```python
from build123d import *

# Parameters (mm, degrees)
SKETCH_2_W          = 65
SKETCH_2_H          = 29
EXTRUDE_1_DEPTH     = 24
FILLET_1_R          = 2
SKETCH_3_R          = 1
CUT_EXTRUDE_1_DEPTH = 6
SKETCH_4_R          = 8
EXTRUDE_2_DEPTH     = 1
FILLET_2_R          = 1
SKETCH_5_R          = 4
EXTRUDE_3_DEPTH     = 6
SKETCH_6_R          = 1
CUT_EXTRUDE_2_DEPTH = 6
EXTRUDE_START       = 1
SKETCH_7_R          = 8
EXTRUDE_4_DEPTH     = 1
FILLET_3_R          = 1
SKETCH_8_R          = 3.5
EXTRUDE_5_DEPTH     = 0.3
SKETCH_9_R          = 3
EXTRUDE_6_DEPTH     = 5.5
SKETCH_10_R         = 1
CUT_EXTRUDE_3_DEPTH = 5.5
SKETCH_11_W         = 6.5
SKETCH_11_H         = 3
EXTRUDE_7_DEPTH     = 1
SKETCH_12_R         = 1.5
CUT_EXTRUDE_4_DEPTH = 6


with BuildPart() as part:
    # ｽｹｯﾁ2 → ﾎﾞｽ - 押し出し1 (new, symmetric)
    with BuildSketch(Plane(origin=(0, 0, 0), x_dir=(1, 0, 0), z_dir=(0, 1, 0))):
        Rectangle(SKETCH_2_W, SKETCH_2_H)
    extrude(amount=EXTRUDE_1_DEPTH, both=True)

    # ﾌｨﾚｯﾄ1
    fillet_1_edges = [part.edges().sort_by_distance(p)[0] for p in [
        (32.5, 0, 14.5),
        (-32.5, 0, 14.5),
        (-32.5, 0, -14.5),
        (32.5, 0, -14.5),
    ]]
    fillet(fillet_1_edges, radius=FILLET_1_R)

    # ｽｹｯﾁ3 → ｶｯﾄ - 押し出し1 (cut)
    with BuildSketch(Plane(origin=(0, 24, 0), x_dir=(1, 0, 0), z_dir=(0, 1, 0))):
        with Locations(Location((-29.5, 0, 0), (0, 0, 270))):
            Circle(SKETCH_3_R)
        with Locations(Location((-17.5, -13, 0), (0, 0, 270))):
            Circle(SKETCH_3_R)
        with Locations(Location((-17.5, 13, 0), (0, 0, 90))):
            Circle(SKETCH_3_R)
    extrude(amount=-CUT_EXTRUDE_1_DEPTH, mode=Mode.SUBTRACT)

    # ｽｹｯﾁ4 → ﾎﾞｽ - 押し出し2 (add)
    with BuildSketch(Plane(origin=(0, 24, 0), x_dir=(1, 0, 0), z_dir=(0, 1, 0))):
        with Locations(Location((20, 0, 0), (0, 0, 270))):
            Circle(SKETCH_4_R)
    extrude(amount=EXTRUDE_2_DEPTH)

    # ﾌｨﾚｯﾄ2
    fillet_2_edges = [part.edges().sort_by_distance(p)[0] for p in [
        (20, 24, -8),
    ]]
    fillet(fillet_2_edges, radius=FILLET_2_R - 0.0001)  # a hair under: the kernel refuses the full size

    # ｽｹｯﾁ5 → ﾎﾞｽ - 押し出し3 (add)
    with BuildSketch(Plane(origin=(0, 25, 0), x_dir=(1, 0, 0), z_dir=(0, 1, 0))):
        with Locations(Location((20, 0, 0), (0, 0, 270))):
            Circle(SKETCH_5_R)
    extrude(amount=EXTRUDE_3_DEPTH)

    # ｽｹｯﾁ6 → ｶｯﾄ - 押し出し2 (cut)
    with BuildSketch(Plane.XZ.offset(24)):
        with Locations(Location((-29.5, 13, 0), (0, 0, 270))):
            Circle(SKETCH_6_R)
        with Locations(Location((-29.5, -13, 0), (0, 0, 90))):
            Circle(SKETCH_6_R)
        with Locations(Location((29.5, -13, 0), (0, 0, 270))):
            Circle(SKETCH_6_R)
        with Locations(Location((29.5, 13, 0), (0, 0, 90))):
            Circle(SKETCH_6_R)
        with Locations(Location((-5.5, 13, 0), (0, 0, 270))):
            Circle(SKETCH_6_R)
        with Locations(Location((-5.5, -13, 0), (0, 0, 90))):
            Circle(SKETCH_6_R)
    extrude(amount=-CUT_EXTRUDE_2_DEPTH, mode=Mode.SUBTRACT)

    # ｽｹｯﾁ7 → ﾎﾞｽ - 押し出し4 (add)
    with BuildSketch(Plane.XZ.offset(24).offset(EXTRUDE_START)):
        with Locations(Location((20, 0, 0), (0, 0, 90))):
            Circle(SKETCH_7_R)
    extrude(amount=-EXTRUDE_4_DEPTH)

    # ﾌｨﾚｯﾄ3
    fillet_3_edges = [part.edges().sort_by_distance(p)[0] for p in [
        (20, -24, -8),
    ]]
    fillet(fillet_3_edges, radius=FILLET_3_R - 0.0001)  # a hair under: the kernel refuses the full size

    # ｽｹｯﾁ8 → ﾎﾞｽ - 押し出し5 (add)
    with BuildSketch(Plane.XZ.offset(25)):
        with Locations(Location((20, 0, 0), (0, 0, 270))):
            Circle(SKETCH_8_R)
    extrude(amount=EXTRUDE_5_DEPTH)

    # ｽｹｯﾁ9 → ﾎﾞｽ - 押し出し6 (add)
    with BuildSketch(Plane.XZ.offset(25)):
        with Locations(Location((20, 0, 0), (0, 0, 270))):
            Circle(SKETCH_9_R)
    extrude(amount=EXTRUDE_6_DEPTH)

    # ｽｹｯﾁ10 → ｶｯﾄ - 押し出し3 (cut)
    with BuildSketch(Plane.XZ.offset(30.5)):
        with Locations(Location((20, 0, 0), (0, 0, 270))):
            Circle(SKETCH_10_R)
    extrude(amount=-CUT_EXTRUDE_3_DEPTH, mode=Mode.SUBTRACT)

    # ｽｹｯﾁ11 → ﾎﾞｽ - 押し出し7 (add)
    with BuildSketch(Plane(origin=(32.5, 0, 0), x_dir=(0, 0, -1), z_dir=(1, 0, 0))):
        with Locations((0, -15.5)):
            Rectangle(SKETCH_11_W, SKETCH_11_H)
    extrude(amount=EXTRUDE_7_DEPTH)

    # ｽｹｯﾁ12 → ｶｯﾄ - 押し出し4 (cut)
    with BuildSketch(Plane(origin=(0, 31, 0), x_dir=(1, 0, 0), z_dir=(0, 1, 0))):
        with Locations(Location((20, 0, 0), (0, 0, 270))):
            Circle(SKETCH_12_R)
    extrude(amount=-CUT_EXTRUDE_4_DEPTH, mode=Mode.SUBTRACT)


solid = part.part
```
Read the model definition and answer for the solid it produces. Units are mm, in the model's axes. A direction names the side the tool comes from. Coordinates: 2 decimals unless noted, no trailing zeros. Order: outer loops, then holes, each group sorted by start corner. A loop starts at its lowest first (then second) coordinate and runs counter-clockwise, first axis right, second up. Notation, with made-up numbers: (87, 64) - (126, 64) arc R35 cw to (126, 97) - close; hole circle Ø7 at (-37.75, -18.75). An arc over 180 degrees is marked (long way). Answer as a JSON object with one key per item and string values. Group by question number.
Item 1: Section A-A (x = -29.5) is taken. Give the vertices of the cut face in (y, z).
Item 2: Flat-ended cylindrical pins translate along their axes: P1, Ø0.5, axis at x = 33, z = 1, coming from the -Y side; P2, Ø1.6, axis at x = -29.5, z = 0, coming from the -Y side; P3, Ø7.5, axis at x = 19.5, z = 0.5, coming from the -Y side; P4, Ø0.6, axis at x = 29.5, z = -13, coming from the -Y side. Find the tip coordinate at first contact, or state that the pin passes through.
Item 3: A tool of negligible diameter and unlimited length cuts with its end or side. For faces 4 (the face through (-6, -18, -13)), 5 (the face through (33.5, -15, 0)), 6 (the face through (-18.39, 21.04, 13.46)), from which of +Z, -Z, +X, -X, +Y, -Y can it reach the whole face along a straight path? Write none if from no direction.
Item 4: Section C-C (x = -17.5) is taken. Give the vertices of the cut face in (y, z), plus the area to 3 significant figures.
Item 5: Section B-B (y = 6) is taken. Give the vertices of the cut face in (x, z).
Item 6: The mould has two halves that part along Z. Classify faces 1 (the face through (-30.49, -21.04, -13.13)), 2 (the face through (23.966, 27.958, -0.521)), 3 (the face through (21, -30.5, 1)): +Z half, -Z half, draft (parallel to the pull), parting line (faces both ways), or undercut.
Item 7: Consider probe 1 along X at (y, z) = (28.2, 0); probe 2 along X at (y, z) = (-21.5, 13); probe 3 along Z at (x, y) = (29, -22). Determine where each line is inside the solid, lowest interval first. Write a range as from..to.
Results are:
{
 "1": {"outline": "(-24, -14.5) - (24, -14.5) - (24, -1) - (18, -1) - (18, 1) - (24, 1) - (24, 14.5) - (-24, 14.5) - (-24, 14) - (-18, 14) - (-18, 12) - (-24, 12) - (-24, -12) - (-18, -12) - (-18, -14) - (-24, -14) - close"},
 "2": {"P1": "stops at y = -17", "P2": "stops at y = -24", "P3": "stops at y = -30.5", "P4": "stops at y = -18"},
 "3": {"face 4": "-Y", "face 5": "+Z, -Z, +X, +Y, -Y", "face 6": "+Y"},
 "4": {"outline": "(-24, -14.5) - (24, -14.5) - (24, -14) - (18, -14) - (18, -12) - (24, -12) - (24, 12) - (18, 12) - (18, 14) - (24, 14) - (24, 14.5) - (-24, 14.5) - close", "area": "1,370 mm^2"},
 "5": {"outline": "(-32.5, -12.5) arc R2 ccw to (-30.5, -14.5) - (30.5, -14.5) arc R2 ccw to (32.5, -12.5) - (32.5, 12.5) arc R2 ccw to (30.5, 14.5) - (-30.5, 14.5) arc R2 ccw to (-32.5, 12.5) - close"},
 "6": {"face 1": "undercut", "face 2": "parting line", "face 3": "draft"},
 "7": {"probe 1": "x = 16..18.5, 21.5..24", "probe 2": "x = -32.44..-30.5, -28.5..-6.5, -4.5..28.5, 30.5..32.44", "probe 3": "z = -14.5..-13.87, -12.13..12.13, 13.87..14.5"}
}
